Could you check a few things on this drawing? It's one solid part, dimensions in mm from its lowest x, y, z. Give positions to 0.01 mm unless a question says otherwise; leave off trailing zeros. Loops run counter-clockwise (first coordinate to the right, second up) from the corner with the lowest first, then second, coordinate; pieces in that order, holes last. Notation, with made-up numbers: M 45.25,7 L 51.25,7 A22 ccw 51.25,37 Z; hole C -22,64.25 d3. An arc over 180 degrees is marked long. Answer in a Markdown table with one row per item. Add a question column.
1. If we section it at D-D on x = 6.25: List the corners of the cut face in (y, z) for me.
2. I need wall thicknesses on line 1 along Z through (x, y) = (30.25, 0.8); line 2 along Z through (x, y) = (6.25, 1.3); line 3 along X through (y, z) = (1.95, 26.5). Which ranges of each line are inside material? Lowest first, please. Write a range as from..to.
3. If we section it at C-C on y = 1.65: List the corners of the cut face in (x, z) for me, then the cut area to 3 significant figures.
4. I'm going to push flat-ended pins straight in: pin 1 Ø1 at (x, z) = (46, 33.5) entering from -Y; pin 2 Ø8 at (x, z) = (30.25, 30.25) entering from -Y. Where does each tip first touch, or does it pass through?
5. If we section it at B-B on z = 54.25: List the corners of the cut face in (x, y) for me, then the cut area to 3 significant figures.
6. If we section it at A-A on x = 30.25: List the corners of the cut face in (y, z) for me.
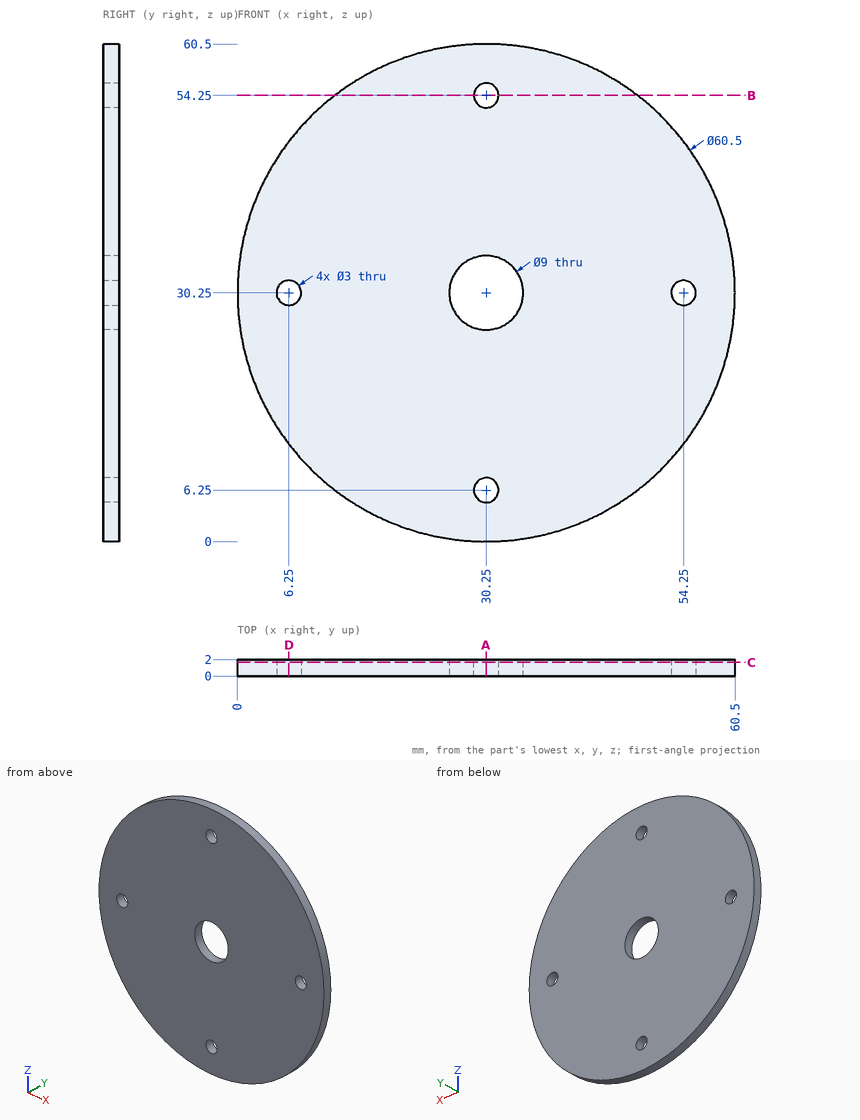
Results:
| question | item | result |
|---|---|---|
| 1 | outline | M 0,11.84 L 2,11.84 L 2,28.75 L 0,28.75 Z; M 0,31.75 L 2,31.75 L 2,48.66 L 0,48.66 Z |
| 2 | line 1 | 0..4.75, 7.75..25.75, 34.75..52.75, 55.75..60.5 |
| 2 | line 2 | 11.84..28.75, 31.75..48.66 |
| 2 | line 3 | 0.23..27.76, 32.74..60.27 |
| 3 | outline | C 30.25,30.25 d60.5; hole C 6.25,30.25 d3; hole C 30.25,30.25 d9; hole C 30.25,6.25 d3; hole C 30.25,54.25 d3; hole C 54.25,30.25 d3 |
| 3 | area | 2,780 mm2 |
| 4 | pin 1 | y = 0 |
| 4 | pin 2 | through |
| 5 | outline | M 11.84,0 L 28.75,0 L 28.75,2 L 11.84,2 Z; M 31.75,0 L 48.66,0 L 48.66,2 L 31.75,2 Z |
| 5 | area | 67.7 mm2 |
| 6 | outline | M 0,0 L 2,0 L 2,4.75 L 0,4.75 Z; M 0,7.75 L 2,7.75 L 2,25.75 L 0,25.75 Z; M 0,34.75 L 2,34.75 L 2,52.75 L 0,52.75 Z; M 0,55.75 L 2,55.75 L 2,60.5 L 0,60.5 Z |
